Work out the finished part from the listing and answer in its coordinate system (mm). A direction names the side the tool comes from. Coordinates: 2 decimals unless noted, no trailing zeros. Loops run counter-clockwise (first coordinate to the right, second up) from the corner with the lowest first, then second, coordinate; pieces in that order, holes last. Notation, with made-up numbers: (27, 46) -> (35, 46) arc R10 ccw to (35, 65) -> close; hole circle Ø11 at (27.25, 42.25). An arc over 180 degrees is marked (long way). Use a Markdown table: item, result. Add a question column.
```python
from build123d import *

# Parameters (mm, degrees)
F0_W     = 95
F0_H     = 95
F0_W_2   = 75
F0_H_2   = 75
F1_DEPTH = 95
F2_W     = 95
F2_H     = 95
F2_W_2   = 75
F2_H_2   = 75
F3_DEPTH = 95
F4_W     = 95
F4_H     = 95
F4_W_2   = 75
F4_H_2   = 75
F5_DEPTH = 95


with BuildPart() as f1:
    # F0 (on Top) → F1 (new body)
    with BuildSketch(Plane.XY):
        Rectangle(F0_W, F0_H)
        Rectangle(F0_W_2, F0_H_2, mode=Mode.SUBTRACT)
    extrude(amount=F1_DEPTH)

    # F2 (on face) → F3 (join)
    with BuildSketch(Plane(origin=(-47.5, 0, 0), x_dir=(0, -1, 0), z_dir=(-1, 0, 0))):
        with Locations((0, 47.5)):
            Rectangle(F2_W, F2_H)
        with Locations((0, 47.5)):
            Rectangle(F2_W_2, F2_H_2, mode=Mode.SUBTRACT)
    extrude(amount=F3_DEPTH)

    # F4 (on face) → F5 (join)
    with BuildSketch(Plane.XZ.offset(47.5)):
        with Locations((0, 47.5)):
            Rectangle(F4_W, F4_H)
        with Locations((0, 47.5)):
            Rectangle(F4_W_2, F4_H_2, mode=Mode.SUBTRACT)
    extrude(amount=F5_DEPTH)


solid = f1.part
```
Item 1: Find the intervals of material crossed by probe 1 along X at (y, z) = (29, 46); probe 2 along Z at (x, y) = (-90, 32.5), in increasing order.
Item 2: Section A-A (y = -29) is taken. Determine the outline of the cut face in (x, z).
Item 3: For faces 5 (the face through (-1, -37.5, 47)), 6 (the face through (-37.5, -94, 47)), 7 (the face through (-47.5, -94, 47)), 8 (the face through (-46, 47.5, 47)), 9 (the face through (-94, 1, 85)), determine the directions among +Z, -Z, +X, -X, +Y, -Y from which every point of the face is accessible in a straight line to the end or side of a thin tool.
Item 4: For a pull along Y with two mould halves and no side action, classify faces 1 (the face through (37.5, -1, 47)), 2 (the face through (-94, -37.5, 47)), 3 (the face through (-43, -142.5, 48)), 4 (the face through (-142.5, 43, 48)) as +Y half, -Y half, draft (parallel to the pull), parting line (faces both ways), or undercut.
Item 5: Given pin 1 (12 mm diameter, centred on x = -114, z = 43, fed in from -Y); pin 2 (1.5 mm diameter, centred on y = -75.5, z = 74, fed in from -X), each flat-ended and moving along its own axis, determine where each tip first touches the part or whether it passes through.
Item 6: Section C-C (y = -61) is taken. Determine the outline of the cut face in (x, z), then the cut area to 3 significant figures.
Item 7: Section B-B (z = 65.5) is taken. Determine the outline of the cut face in (x, y).
Output:
| question | item | result |
|---|---|---|
| 1 | probe 1 | x = -47.5 to -37.5, 37.5 to 47.5 |
| 1 | probe 2 | z = 0 to 10, 85 to 95 |
| 2 | outline | (-142.5, 0) -> (-37.5, 0) -> (-37.5, 95) -> (-142.5, 95) -> (-142.5, 85) -> (-47.5, 85) -> (-47.5, 10) -> (-142.5, 10) -> close; (37.5, 0) -> (47.5, 0) -> (47.5, 95) -> (37.5, 95) -> close |
| 3 | face 5 | +Z, -Z |
| 3 | face 6 | -Y |
| 3 | face 7 | +Z, -Z, -X, -Y |
| 3 | face 8 | +Z, -Z, +X, -X, +Y |
| 3 | face 9 | -X |
| 4 | face 1 | undercut |
| 4 | face 2 | undercut |
| 4 | face 3 | -Y half |
| 4 | face 4 | draft |
| 5 | pin 1 | stops at y = -47.5 |
| 5 | pin 2 | stops at x = -47.5 |
| 6 | outline | (-47.5, 0) -> (47.5, 0) -> (47.5, 95) -> (-47.5, 95) -> close; hole (-37.5, 10) -> (37.5, 10) -> (37.5, 85) -> (-37.5, 85) -> close |
| 6 | area | 3,400 mm2 |
| 7 | outline | (-142.5, -47.5) -> (-47.5, -47.5) -> (-47.5, -142.5) -> (-37.5, -142.5) -> (-37.5, -47.5) -> (37.5, -47.5) -> (37.5, -142.5) -> (47.5, -142.5) -> (47.5, 47.5) -> (-142.5, 47.5) -> (-142.5, 37.5) -> (-47.5, 37.5) -> (-47.5, -37.5) -> (-142.5, -37.5) -> close; hole (-37.5, -37.5) -> (37.5, -37.5) -> (37.5, 37.5) -> (-37.5, 37.5) -> close |
